Source: CAD feature listing. Evaluate the final solid. Frame: model axes, mm. A direction names the side the tool comes from. Give positions to 0.01 mm unless a question says otherwise; leave off trailing zeros. Order: outer loops, then holes, each group sorted by start corner. A loop starts at its lowest first (then second) coordinate and runs counter-clockwise, first axis right, second up. Notation, with made-up numbers: M 42.5,19.25 L 91.5,19.25 A15 cw 91.5,38.25 Z; hole C 53.5,23.5 d5. An arc over 180 degrees is marked long. Use CSV: the item, a comma, the result in double quotes. Start each with the question number.
1. Section query A-A, the plane x = -34.5. Return the cut outline in (y, z), plus the area to 3 significant figures.
2. Pin query (flat end, axial travel): P1, Ø4, axis at x = 26.65, z = -39.5, coming from the -Y side. Return the tip coordinate at first contact, or that it passes through.
3. Mould query, pull axis Z, two halves, no side actions, for faces 1 (the flat face through (24, 1.6, -1)), 2 (the cylindrical face through (-43.832, 0.811, 7.558)). Classes: released by +Z, released by -Z, zero draft, split by the parting line, or undercut.
4. Reachability of faces 3 (the cylindrical face through (-0.327, 0.789, -26.146)), 4 (the flat face through (24, 0, -1)) from +Z, -Z, +X, -X, +Y, -Y: full face, straight path, thin tool, end or side. Return the list, or none.
5. Section query D-D, the plane y = 0.45. State how many separate pieces and enclosed holes the cut face has, plus the area to 3 significant figures.
6. Section query B-B, the plane z = 35.5. Return the cut outline in (x, y), plus the area to 3 significant figures.
7. Section query C-C, the plane x = 10. Return the cut outline in (y, z).
8. Line query: line 1 along Z through (x, y) = (50.5, 1.45); line 2 along X through (y, z) = (0.3, -39.5); line 3 along Z through (x, y) = (42.45, 0.9). Output: solid intervals per line, ascending. Write a range as [from, to].
from build123d import *

# Parameters (mm, degrees)
SKETCH1_W           = 111.7
SKETCH1_H           = 112
BOSS_EXTRUDE1_DEPTH = 1.6
CUT_EXTRUDE1_DEPTH  = 1.6
SKETCH3_R           = 1.675
SKETCH3_R_2         = 1.8
SKETCH3_R_3         = 1.875
CUT_EXTRUDE2_DEPTH  = 1.6


with BuildPart() as part:
    # Sketch1 → Boss-Extrude1 (new body)
    with BuildSketch(Plane(origin=(0, 0, 0), x_dir=(1, 0, 0), z_dir=(0, 1, 0))):
        Rectangle(SKETCH1_W, SKETCH1_H)
        with BuildLine():
            Line((-14.85, -11.3), (-14.85, 11.3))
            ThreePointArc((-14.85, 11.3), (0, 26.15), (14.85, 11.3))
            Line((14.85, 11.3), (14.85, -11.3))
            ThreePointArc((14.85, -11.3), (0, -26.15), (-14.85, -11.3))
        make_face(mode=Mode.SUBTRACT)
    extrude(amount=BOSS_EXTRUDE1_DEPTH)

    # Sketch2 → Cut-Extrude1 (cut)
    with BuildSketch(Plane(origin=(0, 1.6, 0), x_dir=(1, 0, 0), z_dir=(0, 1, 0))):
        with BuildLine():
            Line((2, 47.65), (2, 31.65))
            ThreePointArc((2, 31.65), (0, 29.65), (-2, 31.65))
            Line((-2, 31.65), (-2, 47.65))
            ThreePointArc((-2, 47.65), (0, 49.65), (2, 47.65))
        make_face()
        with BuildLine():
            Line((2, -47.65), (2, -31.65))
            ThreePointArc((2, -31.65), (0, -29.65), (-2, -31.65))
            Line((-2, -31.65), (-2, -47.65))
            ThreePointArc((-2, -47.65), (0, -49.65), (2, -47.65))
        make_face()
    extrude(amount=-CUT_EXTRUDE1_DEPTH, mode=Mode.SUBTRACT)

    # Sketch3 → Cut-Extrude2 (cut)
    with BuildSketch(Plane(origin=(0, 1.6, 0), x_dir=(1, 0, 0), z_dir=(0, 1, 0))):
        with Locations((-50.575, 50.725)):
            Circle(SKETCH3_R)
        with Locations((50.575, 50.725)):
            Circle(SKETCH3_R)
        with Locations((50.575, -50.725)):
            Circle(SKETCH3_R)
        with Locations((-50.575, -50.725)):
            Circle(SKETCH3_R)
        with Locations((-42.65, 39.5)):
            Circle(SKETCH3_R_2)
        with Locations((-26.65, 39.5)):
            Circle(SKETCH3_R_2)
        with Locations((-42.45, -8.825)):
            Circle(SKETCH3_R_3)
        with Locations((-26.45, -8.825)):
            Circle(SKETCH3_R_3)
        with Locations((26.45, -8.825)):
            Circle(SKETCH3_R_3)
        with Locations((42.45, -8.825)):
            Circle(SKETCH3_R_3)
        with Locations((42.65, 39.5)):
            Circle(SKETCH3_R_2)
        with Locations((26.65, 39.5)):
            Circle(SKETCH3_R_2)
        with BuildLine():
            Line((-42.45, 9.3), (-26.45, 9.3))
            ThreePointArc((-26.45, 9.3), (-24.45, 7.3), (-26.45, 5.3))
            Line((-26.45, 5.3), (-42.45, 5.3))
            ThreePointArc((-42.45, 5.3), (-44.45, 7.3), (-42.45, 9.3))
        make_face()
        with BuildLine():
            Line((-42.45, -38.6), (-26.45, -38.6))
            ThreePointArc((-26.45, -38.6), (-24.45, -40.6), (-26.45, -42.6))
            Line((-26.45, -42.6), (-42.45, -42.6))
            ThreePointArc((-42.45, -42.6), (-44.45, -40.6), (-42.45, -38.6))
        make_face()
        with BuildLine():
            Line((-42.45, -22.8), (-26.45, -22.8))
            ThreePointArc((-26.45, -22.8), (-24.45, -24.8), (-26.45, -26.8))
            Line((-26.45, -26.8), (-42.45, -26.8))
            ThreePointArc((-42.45, -26.8), (-44.45, -24.8), (-42.45, -22.8))
        make_face()
        with BuildLine():
            Line((42.45, -38.6), (26.45, -38.6))
            ThreePointArc((26.45, -38.6), (24.45, -40.6), (26.45, -42.6))
            Line((26.45, -42.6), (42.45, -42.6))
            ThreePointArc((42.45, -42.6), (44.45, -40.6), (42.45, -38.6))
        make_face()
        with BuildLine():
            Line((42.45, -22.8), (26.45, -22.8))
            ThreePointArc((26.45, -22.8), (24.45, -24.8), (26.45, -26.8))
            Line((26.45, -26.8), (42.45, -26.8))
            ThreePointArc((42.45, -26.8), (44.45, -24.8), (42.45, -22.8))
        make_face()
        with BuildLine():
            Line((42.45, 9.3), (26.45, 9.3))
            ThreePointArc((26.45, 9.3), (24.45, 7.3), (26.45, 5.3))
            Line((26.45, 5.3), (42.45, 5.3))
            ThreePointArc((42.45, 5.3), (44.45, 7.3), (42.45, 9.3))
        make_face()
    extrude(amount=-CUT_EXTRUDE2_DEPTH, mode=Mode.SUBTRACT)


solid = part.part
Result set:
1,outline,"M 0,-56 L 1.6,-56 L 1.6,-9.3 L 0,-9.3 Z; M 0,-5.3 L 1.6,-5.3 L 1.6,22.8 L 0,22.8 Z; M 0,26.8 L 1.6,26.8 L 1.6,38.6 L 0,38.6 Z; M 0,42.6 L 1.6,42.6 L 1.6,56 L 0,56 Z"
1,area,"160 mm2"
2,P1,"y = 0"
3,face 1,"zero draft"
3,face 2,"undercut"
4,face 3,"+Y, -Y"
4,face 4,"+Z, -Z, +X, -X, -Y"
5,separate pieces,"1"
5,enclosed holes,"21"
5,area,"10,400 mm2"
6,outline,"M -55.85,0 L -2,0 L -2,1.6 L -55.85,1.6 Z; M 2,0 L 55.85,0 L 55.85,1.6 L 2,1.6 Z"
6,area,"172 mm2"
7,outline,"M 0,-56 L 1.6,-56 L 1.6,-22.28 L 0,-22.28 Z; M 0,22.28 L 1.6,22.28 L 1.6,56 L 0,56 Z"
8,line 1,"[-56, -52.4], [-49.05, 49.05], [52.4, 56]"
8,line 2,"[-55.85, -44.45], [-40.85, -28.45], [-24.85, -2], [2, 24.85], [28.45, 40.85], [44.45, 55.85]"
8,line 3,"[-56, -41.29], [-37.71, -9.3], [-5.3, 6.95], [10.7, 22.8], [26.8, 38.6], [42.6, 56]"
